```python
from build123d import *

# Parameters (mm, degrees)
ESBO_O1_R                = 85.4
RESSALTO_EXTRUS_O1_DEPTH = 4
CORTE_EXTRUS_O2_DEPTH    = 5
ESBO_O4_R                = 4
CORTE_EXTRUS_O3_DEPTH    = 5
ESBO_O5_R                = 4.75
CORTE_EXTRUS_O4_DEPTH    = 5
ESBO_O7_R                = 2.1
CORTE_EXTRUS_O5_DEPTH    = 5
CORTE_EXTRUS_O6_REACH    = 6
ESBO_O8_W                = 15
ESBO_O8_H                = 10


with BuildPart() as part:
    # Esboço1 → Ressalto-extrusão1 (new body)
    with BuildSketch(Plane(origin=(0, 0, 0), x_dir=(1, 0, 0), z_dir=(0, 1, 0))):
        Circle(ESBO_O1_R)
    extrude(amount=RESSALTO_EXTRUS_O1_DEPTH)

    # Esboço3 → Corte-extrusão2 (cut, through all)
    with BuildSketch(Plane.XZ):
        with BuildLine():
            Line((6.077686218, 34.468271355), (11.634427904, 65.982119452))
            ThreePointArc((11.634427904, 65.982119452), (0, 67), (-11.634427904, 65.982119452))
            Line((-11.634427904, 65.982119452), (-6.077686218, 34.468271355))
            ThreePointArc((-6.077686218, 34.468271355), (0, 35), (6.077686218, 34.468271355))
        make_face()
    extrude(amount=-CORTE_EXTRUS_O2_DEPTH, mode=Mode.SUBTRACT)

    # Esboço4 → Corte-extrusão3 (cut, through all)
    with BuildSketch(Plane(origin=(0, 4, 0), x_dir=(1, 0, 0), z_dir=(0, 1, 0))):
        with Locations((42.850936979, -24.74)):
            Circle(ESBO_O4_R)
        with Locations((0, 49.48)):
            Circle(ESBO_O4_R)
        with Locations((-42.850936979, -24.74)):
            Circle(ESBO_O4_R)
    extrude(amount=-CORTE_EXTRUS_O3_DEPTH, mode=Mode.SUBTRACT)

    # Esboço5 → Corte-extrusão4 (cut, through all)
    with BuildSketch(Plane.XZ):
        Circle(ESBO_O5_R)
    extrude(amount=-CORTE_EXTRUS_O4_DEPTH, mode=Mode.SUBTRACT)

    # Esboço7 → Corte-extrusão5 (cut, through all)
    with BuildSketch(Plane(origin=(0, 4, 0), x_dir=(1, 0, 0), z_dir=(0, 1, 0))):
        with Locations((-17.5, 8)):
            Circle(ESBO_O7_R)
        with Locations((17.5, 8)):
            Circle(ESBO_O7_R)
        with BuildLine():
            Line((-22, -22), (-19, -22))
            ThreePointArc((-19, -22), (-16, -25), (-19, -28))
            Line((-19, -28), (-22, -28))
            ThreePointArc((-22, -28), (-25, -25), (-22, -22))
        make_face()
        with BuildLine():
            Line((19, -28), (22, -28))
            ThreePointArc((22, -28), (25, -25), (22, -22))
            Line((22, -22), (19, -22))
            ThreePointArc((19, -22), (16, -25), (19, -28))
        make_face()
    extrude(amount=-CORTE_EXTRUS_O5_DEPTH, mode=Mode.SUBTRACT)

    # Esboço8 → Corte-extrusão6 (cut, up to next)
    with BuildSketch(Plane(origin=(0, 4, 0), x_dir=(1, 0, 0), z_dir=(0, 1, 0)), mode=Mode.PRIVATE) as corte_extrus_o6_sk1:
        with Locations((47.5, 29.48)):
            Rectangle(ESBO_O8_W, ESBO_O8_H)
    corte_extrus_o6_tool1 = extrude(corte_extrus_o6_sk1.sketch, amount=-CORTE_EXTRUS_O6_REACH, mode=Mode.PRIVATE) & part.part
    add(corte_extrus_o6_tool1.solids().sort_by_distance((47.5, 4, -29.48))[0], mode=Mode.SUBTRACT)


solid = part.part
```
Here's how the part is built. I have some questions about the finished solid (model axes, mm). Coordinates: 2 decimals unless noted, no trailing zeros. Order: outer loops, then holes, each group sorted by start corner. A loop starts at its lowest first (then second) coordinate and runs counter-clockwise, first axis right, second up. Notation, with made-up numbers: M 44,29.25 L 50,29.25 A17 ccw 50,39.25 Z; hole C 72.25,16 d7. An arc over 180 degrees is marked long. Answer as a JSON object with one key per item and string values. Group by question number.
(1) For pin 1 (1 mm diameter, centred on x = 31, y = 3.5, fed in from -Z); pin 2 (7 mm diameter, centred on x = -42.85, z = 24.74, fed in from +Y); pin 3 (2 mm diameter, centred on y = 1.5, z = -28.5, fed in from +X); pin 4 (2 mm diameter, centred on x = 50.5, y = 3, fed in from -Z), each with a flat end and sliding along its axis, tell me the tip position at first contact or that it passes through.
(2) Suppose I cut it at D-D, the plane x = 31. Please give me the cut outline in (y, z), then the cut area to 3 significant figures.
(3) Suppose I cut it at A-A, the plane z = 0. Please give me the cut outline in (x, y), then the cut area to 3 significant figures.
(4) I need wall thicknesses on probe 1 along Z at (x, y) = (50.5, 0.65); probe 2 along X at (y, z) = (1.65, -8); probe 3 along X at (y, z) = (3.15, 2). Which ranges of each line are inside material? Lowest first, please.
(5) Suppose I cut it at B-B, the plane y = 2. State how many separate pieces and enclosed holes the cut face has, then the cut area to 3 significant figures.
(6) Suppose I cut it at C-C, the plane z = -30.5. Please give me the cut outline in (x, y), then the cut area to 3 significant figures.
(7) If we mould it in two halves opening along Z, with no side actions, what happens to faces 1 (the face through (55, 2, -29)), 2 (the face through (18, 0, -1)), 3 (the face through (-18.51, 1.97, 83.37))? For each: released by +Z, released by -Z, zero draft, split by the parting line, or undercut.
Values found:
{
 "1": {"pin 1": "stops at z = -79.77", "pin 2": "passes through", "pin 3": "stops at x = 80.85", "pin 4": "stops at z = -69.59"},
 "2": {"outline": "M 0,-79.57 L 4,-79.57 L 4,79.57 L 0,79.57 Z", "area": "637 mm^2"},
 "3": {"outline": "M -85.4,0 L -4.75,0 L -4.75,4 L -85.4,4 Z; M 4.75,0 L 85.4,0 L 85.4,4 L 4.75,4 Z", "area": "645 mm^2"},
 "4": {"probe 1": "z = -68.87 to -34.48, -24.48 to 68.87", "probe 2": "x = -85.02 to -19.6, -15.4 to 15.4, 19.6 to 85.02", "probe 3": "x = -85.38 to -4.31, 4.31 to 85.38"},
 "5": {"separate pieces": "1", "enclosed holes": "10", "area": "21,900 mm^2"},
 "6": {"outline": "M -79.77,0 L 40,0 L 40,4 L -79.77,4 Z; M 55,0 L 79.77,0 L 79.77,4 L 55,4 Z", "area": "578 mm^2"},
 "7": {"face 1": "undercut", "face 2": "zero draft", "face 3": "split by the parting line"}
}
